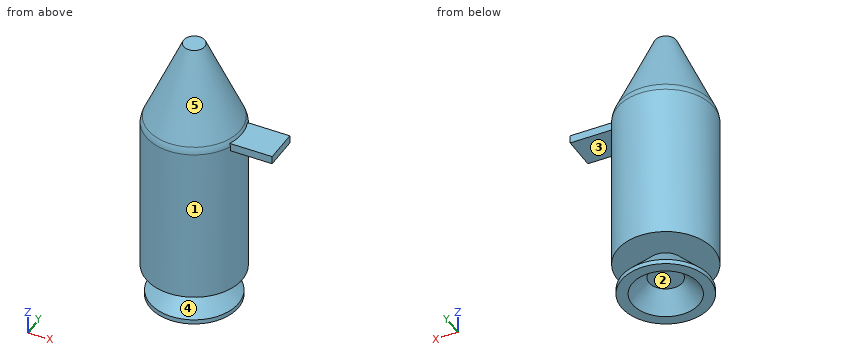
```python
from build123d import *

# Parameters (mm, degrees)
F2_W     = 7.128102
F2_H     = 1.654645
F3_DEPTH = 18


with BuildPart() as f1:
    # F0 (on Front) → F1 (revolve)
    with BuildSketch(Plane.XZ):
        with BuildLine():
            Line((0, 30.909854), (-2.205052, 30.909854))
            Line((-2.205052, 30.909854), (-9.606381, 14.085311))
            ThreePointArc((-9.606381, 14.085311), (-9.859412, 13.365584), (-10, 12.615739))
            Line((-10, 12.615739), (-10, -20.428332))
            Line((-10, -20.428332), (-3.521215, -20.428332))
            Line((-3.521215, -20.428332), (-9.191453, -26.291605))
            Line((-9.191453, -26.291605), (-9.191453, -27.253969))
            Line((-9.191453, -27.253969), (-6.950572, -27.253969))
            Line((-6.950572, -27.253969), (-3.461232, -23.483038))
            Line((-3.461232, -23.483038), (0, -23.483038))
            Line((0, -23.483038), (0, 30.909854))
        make_face()
    revolve(axis=Axis((0, 0, 3.713408), (0, 0, -1)))

    # F2 (on Right) → F3 (join)
    with BuildSketch(Plane.YZ):
        with Locations((0, 12.470122)):
            Rectangle(F2_W, F2_H)
    extrude(amount=F3_DEPTH)


solid = f1.part
```
The model under review builds one solid part; all positions refer to its coordinate system, in mm. Face numbers are marked on the shaded views. A direction names the side the tool comes from. Give positions to 0.01 mm unless a question says otherwise; leave off trailing zeros. Write each loop counter-clockwise with the first axis right and the second up, starting at its lowest first coordinate (ties: lowest second). Pieces come first, ordered by that corner, then holes.
(1) The part is to be moulded in two halves that separate along Y. For the marked faces 1, 2 and 3, say which applies: released by +Y, released by -Y, zero draft, split by the parting line, or undercut.
(2) For P1, Ø0.5, axis at x = 13.5, z = 12.5, coming from the -Y side; P2, Ø2, axis at x = 15, y = -1, coming from the -Z side; P3, Ø1.5, axis at x = 1, z = -19.5, coming from the -Y side; P4, Ø6, axis at y = 2, z = -11.5, coming from the -X side, all flat-tipped, find the tip position at first contact; note any pin that passes through.
(3) To check wall thickness, follow L1, parallel to Z at x = 8.75, y = -2.5; L2, parallel to Z at x = 6.75, y = -5.75; L3, parallel to Y at x = -2.75, z = -12. State the ranges of each line that lie inside material, in increasing order.
(4) Consider section B-B, the plane x = 0. Give the boundary of the cut face in (y, z).
(5) Consider section A-A, the plane z = 8.5. Give the boundary of the cut face in (x, y), and give its area (3 significant figures).
(6) Consider section D-D, the plane z = 19.5. Give the boundary of the cut face in (x, y).
(7) Tool access review of the marked faces 4 and 5: name each direction out of +Z, -Z, +X, -X, +Y, -Y from which nothing blocks a thin tool from reaching the whole face with its end or side.
(8) Consider section C-C, the plane y = 0. Give the boundary of the cut face in (x, z), and give its area (3 significant figures).
Returned:
1. face 1: split by the parting line
1. face 2: undercut
1. face 3: zero draft
2. P1: stops at y = -3.56
2. P2: stops at z = 11.64
2. P3: stops at y = -10
2. P4: stops at x = -10
3. L1: z = -27.25 to -26.2, -20.43 to 15.24
3. L2: z = -27.25 to -25.96, -20.43 to 15.77
3. L3: y = -9.61 to 9.61
4. outline: (-10, -20.43) - (-3.52, -20.43) - (-9.19, -26.29) - (-9.19, -27.25) - (-6.95, -27.25) - (-3.46, -23.48) - (3.46, -23.48) - (6.95, -27.25) - (9.19, -27.25) - (9.19, -26.29) - (3.52, -20.43) - (10, -20.43) - (10, 12.62) arc R5 ccw to (9.61, 14.09) - (2.21, 30.91) - (-2.21, 30.91) - (-9.61, 14.09) arc R5 ccw to (-10, 12.62) - close
5. outline: circle Ø20 at (0, 0)
5. area: 314 mm2
6. outline: circle Ø14.45 at (0, 0)
7. face 4: none
7. face 5: +Z
8. outline: (-10, -20.43) - (-3.52, -20.43) - (-9.19, -26.29) - (-9.19, -27.25) - (-6.95, -27.25) - (-3.46, -23.48) - (3.46, -23.48) - (6.95, -27.25) - (9.19, -27.25) - (9.19, -26.29) - (3.52, -20.43) - (10, -20.43) - (10, 11.64) - (18, 11.64) - (18, 13.3) - (9.88, 13.3) arc R5 ccw to (9.61, 14.09) - (2.21, 30.91) - (-2.21, 30.91) - (-9.61, 14.09) arc R5 ccw to (-10, 12.62) - close
8. area: 955 mm2
